```python
from build123d import *

# Parameters (mm, degrees)
SKETCH005_R      = 1.7
EXTRUDE003_DEPTH = 18
EXTRUDE002_DEPTH = 18
CHAMFER001_SIZE  = 1


with BuildPart() as screw_holes001:
    # Sketch005 → Extrude003 (new body)
    with BuildSketch(Plane.XY):
        with Locations((-51, 61)):
            Circle(SKETCH005_R)
        with Locations((51, 61)):
            Circle(SKETCH005_R)
        with Locations((51, -61)):
            Circle(SKETCH005_R)
        with Locations((-51, -61)):
            Circle(SKETCH005_R)
    extrude(amount=EXTRUDE003_DEPTH)


with BuildPart() as magnet_plate_with_screw_holes001:
    # Sketch004 → Extrude002 (new body)
    with BuildSketch(Plane.XY):
        with BuildLine():
            Line((-57, 63), (-57, -63))
            ThreePointArc((-57, -63), (-55.828427, -65.828427), (-53, -67))
            Line((-53, -67), (53, -67))
            ThreePointArc((53, -67), (55.828427, -65.828427), (57, -63))
            Line((57, -63), (57, 63))
            ThreePointArc((57, 63), (55.828427, 65.828427), (53, 67))
            Line((53, 67), (-53, 67))
            ThreePointArc((-53, 67), (-55.828427, 65.828427), (-57, 63))
        make_face()
    extrude(amount=EXTRUDE002_DEPTH)

    # Cut002: cut screw holes001
    add(screw_holes001.part, mode=Mode.SUBTRACT)

    # Chamfer001
    chamfer001_edges = [magnet_plate_with_screw_holes001.edges().sort_by_distance(p)[0] for p in [
        (0, -67, 0),
        (-52.7, -61, 0),
        (49.3, -61, 0),
        (-52.7, 61, 0),
        (49.3, 61, 0),
        (0, 67, 18),
        (-52.7, -61, 18),
        (49.3, -61, 18),
        (-52.7, 61, 18),
        (49.3, 61, 18),
    ]]
    chamfer(chamfer001_edges, length=CHAMFER001_SIZE)


solid = magnet_plate_with_screw_holes001.part
```
For this review, take the finished solid that the model builds, in its own axes (mm). Round coordinates to 2 decimals unless told otherwise and drop trailing zeros. Order: outer loops, then holes, each group sorted by start corner. A loop starts at its lowest first (then second) coordinate and runs counter-clockwise, first axis right, second up. Notation, with made-up numbers: (-23, 20) -> (18, 20) arc R18 ccw to (18, 30) -> close; hole circle Ø3 at (61, 12.25). An arc over 180 degrees is marked (long way). Use a Markdown table: item, result.
Item 1: Take a section at A-A (y = 61). State the section outline as (x, z) points.
Resolved:
| item | result |
|---|---|
| outline | (-57, 1) -> (-56, 0) -> (-53.7, 0) -> (-52.7, 1) -> (-52.7, 17) -> (-53.7, 18) -> (-56, 18) -> (-57, 17) -> close; (-49.3, 1) -> (-48.3, 0) -> (48.3, 0) -> (49.3, 1) -> (49.3, 17) -> (48.3, 18) -> (-48.3, 18) -> (-49.3, 17) -> close; (52.7, 1) -> (53.7, 0) -> (56, 0) -> (57, 1) -> (57, 17) -> (56, 18) -> (53.7, 18) -> (52.7, 17) -> close |
Item 2: For pin 1 (10 mm diameter, centred on x = -29, y = 46, fed in from -Z); pin 2 (4.5 mm diameter, centred on x = -51, y = 61, fed in from +Z), all flat-tipped, find the tip position at first contact; note any pin that passes through.
Resolved:
| item | result |
|---|---|
| pin 1 | stops at z = 0 |
| pin 2 | stops at z = 17.55 |
Item 3: Draft analysis for pull direction X (two halves, no side actions). For faces 1 (the cylindrical face through (55.797, -65.859, 8.888)), 2 (the cylindrical face through (49.75, 62.15, 8.89)), 3 (the flat face through (-1, 1, 18)), state which applies: +X half, -X half, draft (parallel to the pull), parting line (faces both ways), or undercut.
Resolved:
| item | result |
|---|---|
| face 1 | +X half |
| face 2 | undercut |
| face 3 | draft |
Item 4: Take a section at B-B (x = 51). State the section outline as (y, z) points.
Resolved:
| item | result |
|---|---|
| outline | (-67, 1) -> (-66, 0) -> (-63.7, 0) -> (-62.7, 1) -> (-62.7, 17) -> (-63.7, 18) -> (-66, 18) -> (-67, 17) -> close; (-59.3, 1) -> (-58.3, 0) -> (58.3, 0) -> (59.3, 1) -> (59.3, 17) -> (58.3, 18) -> (-58.3, 18) -> (-59.3, 17) -> close; (62.7, 1) -> (63.7, 0) -> (66, 0) -> (67, 1) -> (67, 17) -> (66, 18) -> (63.7, 18) -> (62.7, 17) -> close |
Item 5: For line 1 along Y through (x, z) = (-51, 8.5), list the stretches that pass through material, from the lowest coordinate up. Write a range as [from, to].
Resolved:
| item | result |
|---|---|
| line 1 | y = [-67, -62.7], [-59.3, 59.3], [62.7, 67] |
